For this review, take the finished solid that the model builds, in its own axes (mm). A direction names the side the tool comes from. Round coordinates to 2 decimals unless told otherwise and drop trailing zeros. Order: outer loops, then holes, each group sorted by start corner. A loop starts at its lowest first (then second) coordinate and runs counter-clockwise, first axis right, second up. Notation, with made-up numbers: (50, 38) -> (70, 38) arc R21 cw to (70, 67) -> close; hole circle Ø3 at (-28, 81.5). An arc over 180 degrees is marked (long way). Use a Markdown table: item, result. Add a question column.
1) Machinability: for faces 4 (the face through (-50, 0, 5)), 5 (the face through (-10.3, -46.37, 8.63)), 6 (the face through (-48, 51, 5)), which of the approach directions +Z, -Z, +X, -X, +Y, -Y give a long, thin tool a straight path to every point of the face, cutting with its end or side? Answer none if there is none.
2) Consider section A-A (y = 15). State the section outline as (x, z) points.
3) Wall thickness on line 1 along Y through (x, z) = (0, 10.5); line 2 along Y through (x, z) = (11.5, 6.75); line 3 along X through (y, z) = (-38.5, 16.5): over which ranges is each line inside the solid? List them lowest first. Write a range as [from, to].
4) Consider section B-B (z = 7.25). State the section outline as (x, y) points.
5) Draft analysis for pull direction Y (two halves, no side actions). For faces 1 (the face through (-6.44, 49.08, 11.16)), 2 (the face through (28.84, -55.45, 10.57)), 3 (the face through (47, 51, 5)), state which applies: pulls with the +Y half, pulls with the -Y half, needs draft (parallel to the pull), parting line crosses it, or undercut.
6) Consider section D-D (y = 30). State the section outline as (x, z) points, plus the area to 3 significant figures.
7) Clearance check with flat-ended pins moving along their axes: P1, Ø1.5, axis at x = -44.5, y = -31, coming from the +Z side; P2, Ø5, axis at x = -21, y = 46, coming from the +Z side; P3, Ø4, axis at y = -48.5, z = 4.5, coming from the -X side; P4, Ø2, axis at x = 14, z = 15.5, coming from the -Y side. State where each tip first meets the part, or that it passes through.
8) Consider section C-C (y = -8.5). State the section outline as (x, z) points, plus the area to 3 significant figures.
```python
from build123d import *

# Parameters (mm, degrees)
F0_R     = 47.5
F1_DEPTH = 5
F2_R     = 62.5
F2_R_2   = 60.5
F2_R_3   = 49.5
F2_R_4   = 47.5
F3_DEPTH = 12.5


with BuildPart() as f1:
    # F0 (on Top) → F1 (new body)
    with BuildSketch(Plane.XY):
        with BuildLine():
            ThreePointArc((-7.47e-08, 62.5), (-44.1941738506, 44.1941737978), (-62.5, 0))
            ThreePointArc((-62.5, 0), (0, -62.5), (62.5, 0))
            ThreePointArc((62.5, 0), (44.1941737978, 44.1941738506), (-7.47e-08, 62.5))
        make_face()
        Circle(F0_R, mode=Mode.SUBTRACT)
        with BuildLine():
            Line((-62.5, 63.5), (-62.5, 0))
            ThreePointArc((-62.5, 0), (-44.1941738506, 44.1941737978), (-7.47e-08, 62.5))
            add(Edge.make_bspline(
                [(-62.5, 63.5), (-41.6666666667, 63), (-20.8333333333, 62.5), (0, 62.5)],
                knots=[0, 0, 0, 0, 0.5, 0.5, 0.5, 0.5], degree=3))
        make_face()
        with BuildLine():
            ThreePointArc((-7.47e-08, 62.5), (44.1941737978, 44.1941738506), (62.5, 0))
            Line((62.5, 0), (62.5, 63.5))
            add(Edge.make_bspline(
                [(0, 62.5), (20.8333333333, 62.5), (41.6666666667, 63), (62.5, 63.5)],
                knots=[0.5, 0.5, 0.5, 0.5, 1, 1, 1, 1], degree=3))
        make_face()
    extrude(amount=F1_DEPTH)

    # F2 (on face) → F3 (join)
    with BuildSketch(Plane.XY.offset(5)):
        Circle(F2_R)
        Circle(F2_R_2, mode=Mode.SUBTRACT)
        Circle(F2_R_3)
        Circle(F2_R_4, mode=Mode.SUBTRACT)
    extrude(amount=F3_DEPTH)


solid = f1.part
```
Results list:
| question | item | result |
|---|---|---|
| 1 | face 4 | +Z |
| 1 | face 5 | +Z, -Z |
| 1 | face 6 | +Z, -X, +Y |
| 2 | outline | (-62.5, 0) -> (-45.07, 0) -> (-45.07, 17.5) -> (-47.17, 17.5) -> (-47.17, 5) -> (-58.61, 5) -> (-58.61, 17.5) -> (-60.67, 17.5) -> (-60.67, 5) -> (-62.5, 5) -> close; (45.07, 0) -> (62.5, 0) -> (62.5, 5) -> (60.67, 5) -> (60.67, 17.5) -> (58.61, 17.5) -> (58.61, 5) -> (47.17, 5) -> (47.17, 17.5) -> (45.07, 17.5) -> close |
| 3 | line 1 | [-62.5, -60.5], [-49.5, -47.5], [47.5, 49.5], [60.5, 62.5] |
| 3 | line 2 | [-61.43, -59.4], [-48.15, -46.09], [46.09, 48.15], [59.4, 61.43] |
| 3 | line 3 | [-49.23, -46.67], [-31.11, -27.82], [27.82, 31.11], [46.67, 49.23] |
| 4 | outline | circle Ø125 at (0, 0); circle Ø99 at (0, 0); hole circle Ø121 at (0, 0); hole circle Ø95 at (0, 0) |
| 5 | face 1 | undercut |
| 5 | face 2 | parting line crosses it |
| 5 | face 3 | needs draft |
| 6 | outline | (-62.5, 0) -> (-36.83, 0) -> (-36.83, 17.5) -> (-39.37, 17.5) -> (-39.37, 5) -> (-52.54, 5) -> (-52.54, 17.5) -> (-54.83, 17.5) -> (-54.83, 5) -> (-62.5, 5) -> close; (36.83, 0) -> (62.5, 0) -> (62.5, 5) -> (54.83, 5) -> (54.83, 17.5) -> (52.54, 17.5) -> (52.54, 5) -> (39.37, 5) -> (39.37, 17.5) -> (36.83, 17.5) -> close |
| 6 | area | 378 mm2 |
| 7 | P1 | z = 5 |
| 7 | P2 | z = 17.5 |
| 7 | P3 | x = -41.76 |
| 7 | P4 | y = -61.13 |
| 8 | outline | (-61.92, 0) -> (-46.73, 0) -> (-46.73, 17.5) -> (-48.76, 17.5) -> (-48.76, 5) -> (-59.9, 5) -> (-59.9, 17.5) -> (-61.92, 17.5) -> close; (46.73, 0) -> (61.92, 0) -> (61.92, 17.5) -> (59.9, 17.5) -> (59.9, 5) -> (48.76, 5) -> (48.76, 17.5) -> (46.73, 17.5) -> close |
| 8 | area | 253 mm2 |
